from build123d import *

# Parameters (mm, degrees)
SKETCH2_W           = 30
SKETCH2_H           = 60
SKETCH2_R           = 1.6
SKETCH2_R_2         = 1.544536525
BOSS_EXTRUDE1_DEPTH = 36
SKETCH3_W           = 30
SKETCH3_H           = 49.856005965
CUT_EXTRUDE1_DEPTH  = 26
SKETCH4_W           = 30
SKETCH4_H           = 12
CUT_EXTRUDE2_DEPTH  = 5
SKETCH5_R           = 3.2
CUT_EXTRUDE3_DEPTH  = 26
SKETCH6_R           = 4
CUT_EXTRUDE4_DEPTH  = 26
SKETCH8_W           = 48
SKETCH8_H           = 36
BOSS_EXTRUDE3_DEPTH = 6
CHAMFER1_SIZE       = 2
FILLET1_R           = 4
FILLET2_R           = 4


with BuildPart() as part:
    # Sketch2 → Boss-Extrude1 (new body)
    with BuildSketch(Plane(origin=(0, 0, 0), x_dir=(1, 0, 0), z_dir=(0, 1, 0))):
        with Locations((15, 30)):
            Rectangle(SKETCH2_W, SKETCH2_H)
        with Locations(Location((3.45, 3, 0), (0, 0, 270))):
            Circle(SKETCH2_R, mode=Mode.SUBTRACT)
        with Locations(Location((22.5, 3, 0), (0, 0, 270))):
            Circle(SKETCH2_R_2, mode=Mode.SUBTRACT)
        with Locations(Location((4, 55, 0), (0, 0, 270))):
            Circle(SKETCH2_R, mode=Mode.SUBTRACT)
        with Locations(Location((22, 55, 0), (0, 0, 270))):
            Circle(SKETCH2_R, mode=Mode.SUBTRACT)
    extrude(amount=BOSS_EXTRUDE1_DEPTH)

    # Sketch3 → Cut-Extrude1 (cut)
    with BuildSketch(Plane(origin=(0, 36, 0), x_dir=(1, 0, 0), z_dir=(0, 1, 0))):
        with Locations((15, 24.928002983)):
            Rectangle(SKETCH3_W, SKETCH3_H)
    extrude(amount=-CUT_EXTRUDE1_DEPTH, mode=Mode.SUBTRACT)

    # Sketch4 → Cut-Extrude2 (cut)
    with BuildSketch(Plane.XZ):
        with Locations((15, -6)):
            Rectangle(SKETCH4_W, SKETCH4_H)
    extrude(amount=-CUT_EXTRUDE2_DEPTH, mode=Mode.SUBTRACT)

    # Sketch5 → Cut-Extrude3 (cut)
    with BuildSketch(Plane(origin=(0, 36, 0), x_dir=(1, 0, 0), z_dir=(0, 1, 0))):
        with Locations(Location((4, 55, 0), (0, 0, 270))):
            Circle(SKETCH5_R)
        with Locations(Location((22, 55, 0), (0, 0, 270))):
            Circle(SKETCH5_R)
    extrude(amount=-CUT_EXTRUDE3_DEPTH, mode=Mode.SUBTRACT)

    # Sketch6 → Cut-Extrude4 (cut)
    with BuildSketch(Plane(origin=(0, 0, -60), x_dir=(-1, 0, 0), z_dir=(0, 0, -1))):
        with Locations((-13, 14)):
            Circle(SKETCH6_R)
    extrude(amount=-CUT_EXTRUDE4_DEPTH, mode=Mode.SUBTRACT)

    # Sketch8 → Boss-Extrude3 (add)
    with BuildSketch(Plane(origin=(30, 0, 0), x_dir=(0, 0, -1), z_dir=(1, 0, 0))):
        with Locations((36, 18)):
            Rectangle(SKETCH8_W, SKETCH8_H)
    extrude(amount=BOSS_EXTRUDE3_DEPTH)

    # Chamfer1
    chamfer1_edges = [part.edges().sort_by_distance(p)[0] for p in [
        (15, 5, -12),
    ]]
    chamfer(chamfer1_edges, length=CHAMFER1_SIZE)

    # Fillet1
    # the kernel refuses this fillet: 4 mm, written as the material it adds along each edge
    with BuildSketch(Plane(origin=(30, 10, -12), x_dir=(0, 0, 1), z_dir=(0, -1, 0))) as fillet1_piece_1_section:
        with BuildLine():
            CenterArc((FILLET1_R, -FILLET1_R), FILLET1_R, 90, 90)
            Line((0, -FILLET1_R), (0, 0))
            Line((0, 0), (FILLET1_R, 0))
        make_face()
    fillet1_piece_1 = extrude(amount=17, mode=Mode.PRIVATE)
    fillet1_piece_1 = split(fillet1_piece_1, bisect_by=Plane(origin=(30.901414649, 5.69775692, -9.30224308), z_dir=(0, 0.7071067811865476, -0.7071067811865476)), keep=Keep.TOP, mode=Mode.PRIVATE)
    add(fillet1_piece_1)
    with BuildSketch(Plane(origin=(30, 20, -12), x_dir=(0, 0, 1), z_dir=(0, -1, 0))) as fillet1_piece_2_section:
        with BuildLine():
            CenterArc((FILLET1_R, -FILLET1_R), FILLET1_R, 90, 90)
            Line((0, -FILLET1_R), (0, 0))
            Line((0, 0), (FILLET1_R, 0))
        make_face()
    fillet1_piece_2 = extrude(amount=27, mode=Mode.PRIVATE)
    fillet1_piece_2 = split(fillet1_piece_2, bisect_by=Plane(origin=(30.104627362, 5, -9.206224594), z_dir=(0, 1, 0)), keep=Keep.TOP, mode=Mode.PRIVATE)
    fillet1_piece_2 = split(fillet1_piece_2, bisect_by=Plane(origin=(30.104627362, 5.595331555, -9.404668445), z_dir=(0, -0.7071067811865476, 0.7071067811865476)), keep=Keep.TOP, mode=Mode.PRIVATE)
    add(fillet1_piece_2)

    # Fillet2
    # the kernel refuses this fillet: 4 mm, written as the material it adds along each edge
    with BuildSketch(Plane(origin=(26, 14, -45.856005965), x_dir=(0, 0, -1), z_dir=(0, -1, 0))) as fillet2_piece_1_section:
        Polygon((0, 0), (FILLET2_R * 1.02, 0), (FILLET2_R * 1.02, FILLET2_R * 1.02), (0, FILLET2_R * 1.02), align=None)
    fillet2_piece_1 = extrude(amount=FILLET2_R * 1.02, mode=Mode.PRIVATE)
    fillet2_piece_1 = fillet2_piece_1 - Plane(origin=(26, 14, -45.856005965), x_dir=(-0.7071067811865475, 0, 0.7071067811865475), z_dir=(0, -1, 0)) * Sphere(FILLET2_R, mode=Mode.PRIVATE)
    add(fillet2_piece_1)
    with BuildSketch(Plane(origin=(26, 10, -49.856005965), x_dir=(0, 1, 0), z_dir=(-1, 0, 0))) as fillet2_piece_2_section:
        with BuildLine():
            CenterArc((FILLET2_R, -FILLET2_R), FILLET2_R, 90, 90)
            Line((0, -FILLET2_R), (0, 0))
            Line((0, 0), (FILLET2_R, 0))
        make_face()
    fillet2_piece_2 = extrude(amount=13, mode=Mode.PRIVATE)
    fillet2_piece_2 = fillet2_piece_2 - Plane(origin=(13, 14, -48.921311945), x_dir=(-1, 0, 0), z_dir=(0, 0, -1)) * Cylinder(4, 42, mode=Mode.PRIVATE)
    add(fillet2_piece_2)
    with BuildSketch(Plane(origin=(30, 36, -49.856005965), x_dir=(-1, 0, 0), z_dir=(0, -1, 0))) as fillet2_piece_3:
        with BuildLine():
            CenterArc((FILLET2_R, -FILLET2_R), FILLET2_R, 90, 90)
            Line((0, -FILLET2_R), (0, 0))
            Line((0, 0), (FILLET2_R, 0))
        make_face()
    extrude(amount=22)
    with BuildSketch(Plane(origin=(13, 10, -49.856005965), x_dir=(0, 1, 0), z_dir=(-1, 0, 0))) as fillet2_piece_4_section:
        with BuildLine():
            CenterArc((FILLET2_R, -FILLET2_R), FILLET2_R, 90, 90)
            Line((0, -FILLET2_R), (0, 0))
            Line((0, 0), (FILLET2_R, 0))
        make_face()
    fillet2_piece_4 = extrude(amount=13, mode=Mode.PRIVATE)
    fillet2_piece_4 = fillet2_piece_4 - Plane(origin=(13, 14, -48.921311944), x_dir=(-1, 0, 0), z_dir=(0, 0, -1)) * Cylinder(4, 43, mode=Mode.PRIVATE)
    add(fillet2_piece_4)
    with BuildSketch(Plane(origin=(30, 10, -12), x_dir=(0, 1, 0), z_dir=(0, 0, -1))) as fillet2_piece_5:
        with BuildLine():
            CenterArc((FILLET2_R, -FILLET2_R), FILLET2_R, 90, 90)
            Line((0, -FILLET2_R), (0, 0))
            Line((0, 0), (FILLET2_R, 0))
        make_face()
    extrude(amount=33.856005965)


solid = part.part
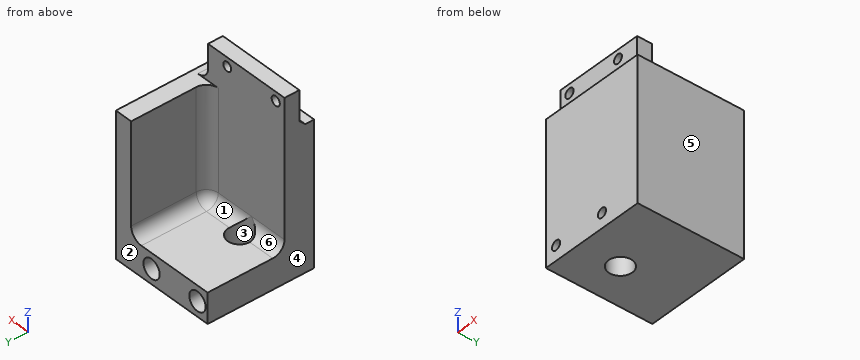
For this review, take the finished solid that the model builds, in its own axes (mm). Face numbers are marked on the shaded views. A direction names the side the tool comes from. Round coordinates to 2 decimals unless told otherwise and drop trailing zeros. Loops run counter-clockwise (first coordinate to the right, second up) from the corner with the lowest first, then second, coordinate; pieces in that order, holes last. Notation, with made-up numbers: (-26.5, 43.25) - (-20.5, 43.25) arc R9 cw to (-20.5, 48.25) - close; hole circle Ø5 at (28.25, 83.5). An arc over 180 degrees is marked (long way). Use one line per item in the form item = value.
Item 1: Consider section B-B on y = 27. Write out the cut boundary in (x, z), then the cut area to 3 significant figures.
Answers:
outline = (0, -60) - (36, -60) - (36, -12) - (30, -12) - (30, -45.86) arc R4 cw to (26, -49.86) - (0, -49.86) - close; hole circle Ø6.4 at (4, -55); hole circle Ø6.4 at (22, -55)
area = 531 mm^2
Item 2: Mouldability with a two-part tool opening along X and no side actions: class the marked faces 3, 4, 5 and 6 as +X half, -X half, draft (parallel to the pull), parting line (faces both ways), or undercut.
Answers:
face_3 = undercut
face_4 = -X half
face_5 = +X half
face_6 = draft
Item 3: Consider section A-A on z = -55. Write out the cut boundary in (x, y), then the cut area to 3 significant figures.
Answers:
outline = (0, 0) - (2.4, 0) - (2.4, 10) - (0.8, 10) - (0.8, 36) - (0, 36) - close; (5.6, 0) - (20.4, 0) - (20.4, 10) - (18.8, 10) - (18.8, 36) - (7.2, 36) - (7.2, 10) - (5.6, 10) - close; (23.6, 0) - (36, 0) - (36, 36) - (25.2, 36) - (25.2, 10) - (23.6, 10) - close; hole circle Ø8 at (13, 14)
area = 849 mm^2
Item 4: Clearance check with flat-ended pins moving along their axes: P1, Ø11, axis at y = 19.5, z = -29.5, coming from the -X side; P2, Ø3, axis at x = 22, z = -55, coming from the -Y side; P3, Ø2.5, axis at y = 6.5, z = -4, coming from the +X side; P4, Ø18, axis at x = 17, y = 21.5, coming from the +Z side. State where each tip first meets the part, or that it passes through.
Answers:
P1 = 30
P2 = through
P3 = 30
P4 = -49.56
Item 5: Tool access review of the marked faces 1 and 2: name each direction out of +Z, -Z, +X, -X, +Y, -Y from which nothing blocks a thin tool from reaching the whole face with its end or side.
Answers:
face_1 = +Z, -X, +Y
face_2 = +Z, -Z, +X, -X, +Y
Item 6: Consider section D-D on x = 33. Write out the cut boundary in (y, z).
Answers:
outline = (0, -60) - (36, -60) - (36, -12) - (10, -12) - (10, -11.87) - (3.13, -11.87) - (3, -12) - (0, -12) - close
Item 7: Consider section C-C on z = -3. Write out the cut boundary in (x, y).
Answers:
outline = (0, 5) - (1.85, 5) - (1.85, 10) - (0, 10) - close; (5.05, 5) - (20.96, 5) - (20.96, 10) - (5.05, 10) - close; (24.04, 5) - (30, 5) - (30, 10) - (24.04, 10) - close
Item 8: For line 1 (Y direction, x = 13, z = -51); line 2 (X direction, y = 7, z = -3); line 3 (X direction, y = 2.5, z = -55), list the stretches that pass through material, from the lowest coordinate up.
Answers:
line_1 = 0 to 10, 18 to 36
line_2 = 0 to 1.85, 5.05 to 20.96, 24.04 to 30
line_3 = 0 to 2.4, 5.6 to 20.4, 23.6 to 36
